```python
from build123d import *

# Parameters (mm, degrees)
CROQUIS1_R              = 2.55
SALIENTE_EXTRUIR1_DEPTH = 400


with BuildPart() as part:
    # Croquis1 → Saliente-Extruir1 (new body)
    with BuildSketch(Plane.XY):
        with BuildLine():
            Line((-20, -9), (-20, -3.95))
            ThreePointArc((-20, -3.95), (-19.912132034, -3.737867966), (-19.7, -3.65))
            Line((-19.7, -3.65), (-19.5, -3.65))
            Line((-19.5, -3.65), (-19.5, -3.15))
            Line((-19.5, -3.15), (-18, -3.15))
            Line((-18, -3.15), (-18, -4.85))
            ThreePointArc((-18, -4.85), (-17.912132034, -5.062132034), (-17.7, -5.15))
            Line((-17.7, -5.15), (-16.5, -5.15))
            Line((-16.5, -5.15), (-14.485786438, -3.135786438))
            ThreePointArc((-14.485786438, -3.135786438), (-14.052240935, -2.48693974), (-13.9, -1.721572875))
            Line((-13.9, -1.721572875), (-13.9, 1.721572875))
            ThreePointArc((-13.9, 1.721572875), (-14.052240935, 2.48693974), (-14.485786438, 3.135786438))
            Line((-14.485786438, 3.135786438), (-16.5, 5.15))
            Line((-16.5, 5.15), (-17.7, 5.15))
            ThreePointArc((-17.7, 5.15), (-17.912132034, 5.062132034), (-18, 4.85))
            Line((-18, 4.85), (-18, 3.15))
            Line((-18, 3.15), (-19.5, 3.15))
            Line((-19.5, 3.15), (-19.5, 3.65))
            Line((-19.5, 3.65), (-19.7, 3.65))
            ThreePointArc((-19.7, 3.65), (-19.912132034, 3.737867966), (-20, 3.95))
            Line((-20, 3.95), (-20, 9))
            ThreePointArc((-20, 9), (-19.707106781, 9.707106781), (-19, 10))
            Line((-19, 10), (-13.95, 10))
            ThreePointArc((-13.95, 10), (-13.737867966, 9.912132034), (-13.65, 9.7))
            Line((-13.65, 9.7), (-13.65, 9.5))
            Line((-13.65, 9.5), (-13.15, 9.5))
            Line((-13.15, 9.5), (-13.15, 8))
            Line((-13.15, 8), (-14.85, 8))
            ThreePointArc((-14.85, 8), (-15.062132034, 7.912132034), (-15.15, 7.7))
            Line((-15.15, 7.7), (-15.15, 6.5))
            Line((-15.15, 6.5), (-13.135786438, 4.485786438))
            ThreePointArc((-13.135786438, 4.485786438), (-12.48693974, 4.052240935), (-11.721572875, 3.9))
            Line((-11.721572875, 3.9), (-8.278427125, 3.9))
            ThreePointArc((-8.278427125, 3.9), (-7.51306026, 4.052240935), (-6.864213562, 4.485786438))
            Line((-6.864213562, 4.485786438), (-4.85, 6.5))
            Line((-4.85, 6.5), (-4.85, 7.7))
            ThreePointArc((-4.85, 7.7), (-4.937867966, 7.912132034), (-5.15, 8))
            Line((-5.15, 8), (-6.85, 8))
            Line((-6.85, 8), (-6.85, 9.5))
            Line((-6.85, 9.5), (-6.35, 9.5))
            Line((-6.35, 9.5), (-6.35, 9.7))
            ThreePointArc((-6.35, 9.7), (-6.262132034, 9.912132034), (-6.05, 10))
            Line((-6.05, 10), (6.05, 10))
            ThreePointArc((6.05, 10), (6.262132034, 9.912132034), (6.35, 9.7))
            Line((6.35, 9.7), (6.35, 9.5))
            Line((6.35, 9.5), (6.85, 9.5))
            Line((6.85, 9.5), (6.85, 8))
            Line((6.85, 8), (5.15, 8))
            ThreePointArc((5.15, 8), (4.937867966, 7.912132034), (4.85, 7.7))
            Line((4.85, 7.7), (4.85, 6.5))
            Line((4.85, 6.5), (6.864213562, 4.485786438))
            ThreePointArc((6.864213562, 4.485786438), (7.51306026, 4.052240935), (8.278427125, 3.9))
            Line((8.278427125, 3.9), (11.721572875, 3.9))
            ThreePointArc((11.721572875, 3.9), (12.48693974, 4.052240935), (13.135786438, 4.485786438))
            Line((13.135786438, 4.485786438), (15.15, 6.5))
            Line((15.15, 6.5), (15.15, 7.7))
            ThreePointArc((15.15, 7.7), (15.062132034, 7.912132034), (14.85, 8))
            Line((14.85, 8), (13.15, 8))
            Line((13.15, 8), (13.15, 9.5))
            Line((13.15, 9.5), (13.65, 9.5))
            Line((13.65, 9.5), (13.65, 9.7))
            ThreePointArc((13.65, 9.7), (13.737867966, 9.912132034), (13.95, 10))
            Line((13.95, 10), (19, 10))
            ThreePointArc((19, 10), (19.707106781, 9.707106781), (20, 9))
            Line((20, 9), (20, 3.95))
            ThreePointArc((20, 3.95), (19.912132034, 3.737867966), (19.7, 3.65))
            Line((19.7, 3.65), (19.5, 3.65))
            Line((19.5, 3.65), (19.5, 3.15))
            Line((19.5, 3.15), (18, 3.15))
            Line((18, 3.15), (18, 4.85))
            ThreePointArc((18, 4.85), (17.912132034, 5.062132034), (17.7, 5.15))
            Line((17.7, 5.15), (16.5, 5.15))
            Line((16.5, 5.15), (14.485786438, 3.135786438))
            ThreePointArc((14.485786438, 3.135786438), (14.052240935, 2.48693974), (13.9, 1.721572875))
            Line((13.9, 1.721572875), (13.9, -1.721572875))
            ThreePointArc((13.9, -1.721572875), (14.052240935, -2.48693974), (14.485786438, -3.135786438))
            Line((14.485786438, -3.135786438), (16.5, -5.15))
            Line((16.5, -5.15), (17.7, -5.15))
            ThreePointArc((17.7, -5.15), (17.912132034, -5.062132034), (18, -4.85))
            Line((18, -4.85), (18, -3.15))
            Line((18, -3.15), (19.5, -3.15))
            Line((19.5, -3.15), (19.5, -3.65))
            Line((19.5, -3.65), (19.7, -3.65))
            ThreePointArc((19.7, -3.65), (19.912132034, -3.737867966), (20, -3.95))
            Line((20, -3.95), (20, -9))
            ThreePointArc((20, -9), (19.707106781, -9.707106781), (19, -10))
            Line((19, -10), (13.65, -10))
            Line((13.65, -10), (13.65, -9.5))
            Line((13.65, -9.5), (13.15, -9.5))
            Line((13.15, -9.5), (13.15, -8))
            Line((13.15, -8), (14.85, -8))
            ThreePointArc((14.85, -8), (15.062132034, -7.912132034), (15.15, -7.7))
            Line((15.15, -7.7), (15.15, -6.5))
            Line((15.15, -6.5), (13.135786438, -4.485786438))
            ThreePointArc((13.135786438, -4.485786438), (12.48693974, -4.052240935), (11.721572875, -3.9))
            Line((11.721572875, -3.9), (8.278427125, -3.9))
            ThreePointArc((8.278427125, -3.9), (7.51306026, -4.052240935), (6.864213562, -4.485786438))
            Line((6.864213562, -4.485786438), (4.85, -6.5))
            Line((4.85, -6.5), (4.85, -7.7))
            ThreePointArc((4.85, -7.7), (4.937867966, -7.912132034), (5.15, -8))
            Line((5.15, -8), (6.85, -8))
            Line((6.85, -8), (6.85, -9.5))
            Line((6.85, -9.5), (6.35, -9.5))
            Line((6.35, -9.5), (6.35, -9.7))
            ThreePointArc((6.35, -9.7), (6.262132034, -9.912132034), (6.05, -10))
            Line((6.05, -10), (0, -10))
            Line((0, -10), (-6.05, -10))
            ThreePointArc((-6.05, -10), (-6.262132034, -9.912132034), (-6.35, -9.7))
            Line((-6.35, -9.7), (-6.35, -9.5))
            Line((-6.35, -9.5), (-6.85, -9.5))
            Line((-6.85, -9.5), (-6.85, -8))
            Line((-6.85, -8), (-5.15, -8))
            ThreePointArc((-5.15, -8), (-4.937867966, -7.912132034), (-4.85, -7.7))
            Line((-4.85, -7.7), (-4.85, -6.5))
            Line((-4.85, -6.5), (-6.864213562, -4.485786438))
            ThreePointArc((-6.864213562, -4.485786438), (-7.51306026, -4.052240935), (-8.278427125, -3.9))
            Line((-8.278427125, -3.9), (-11.721572875, -3.9))
            ThreePointArc((-11.721572875, -3.9), (-12.48693974, -4.052240935), (-13.135786438, -4.485786438))
            Line((-13.135786438, -4.485786438), (-15.15, -6.5))
            Line((-15.15, -6.5), (-15.15, -7.7))
            ThreePointArc((-15.15, -7.7), (-15.062132034, -7.912132034), (-14.85, -8))
            Line((-14.85, -8), (-13.15, -8))
            Line((-13.15, -8), (-13.15, -9.5))
            Line((-13.15, -9.5), (-13.65, -9.5))
            Line((-13.65, -9.5), (-13.65, -9.7))
            ThreePointArc((-13.65, -9.7), (-13.737867966, -9.912132034), (-13.95, -10))
            Line((-13.95, -10), (-19, -10))
            ThreePointArc((-19, -10), (-19.707106781, -9.707106781), (-20, -9))
        make_face()
        with Locations((-10, 0)):
            Circle(CROQUIS1_R, mode=Mode.SUBTRACT)
        with Locations((10, 0)):
            Circle(CROQUIS1_R, mode=Mode.SUBTRACT)
        with BuildLine():
            Line((-6.1, 1.721572875), (-6.1, -1.721572875))
            ThreePointArc((-6.1, -1.721572875), (-5.947759065, -2.48693974), (-5.514213562, -3.135786438))
            Line((-5.514213562, -3.135786438), (-3.5, -5.15))
            Line((-3.5, -5.15), (-0.942893219, -7.707106781))
            ThreePointArc((-0.942893219, -7.707106781), (-0.61846987, -7.923879533), (-0.235786438, -8))
            Line((-0.235786438, -8), (0.235786438, -8))
            ThreePointArc((0.235786438, -8), (0.61846987, -7.923879533), (0.942893219, -7.707106781))
            Line((0.942893219, -7.707106781), (3.5, -5.15))
            Line((3.5, -5.15), (5.514213562, -3.135786438))
            ThreePointArc((5.514213562, -3.135786438), (5.947759065, -2.48693974), (6.1, -1.721572875))
            Line((6.1, -1.721572875), (6.1, 1.721572875))
            ThreePointArc((6.1, 1.721572875), (5.947759065, 2.48693974), (5.514213562, 3.135786438))
            Line((5.514213562, 3.135786438), (3.5, 5.15))
            Line((3.5, 5.15), (0.942893219, 7.707106781))
            ThreePointArc((0.942893219, 7.707106781), (0.61846987, 7.923879533), (0.235786438, 8))
            Line((0.235786438, 8), (-0.235786438, 8))
            ThreePointArc((-0.235786438, 8), (-0.61846987, 7.923879533), (-0.942893219, 7.707106781))
            Line((-0.942893219, 7.707106781), (-3.5, 5.15))
            Line((-3.5, 5.15), (-5.514213562, 3.135786438))
            ThreePointArc((-5.514213562, 3.135786438), (-5.947759065, 2.48693974), (-6.1, 1.721572875))
        make_face(mode=Mode.SUBTRACT)
    extrude(amount=SALIENTE_EXTRUIR1_DEPTH)


solid = part.part
```
Build history of the part. All positions in model axes, mm. Coordinates: 2 decimals unless noted, no trailing zeros.
Item 1: Drop flat-ended pins along their axis: pin 1 Ø1.5 at (x, z) = (9, 277.5) entering from +Y; pin 2 Ø4 at (x, z) = (10, 68) entering from -Y; pin 3 Ø5 at (x, y) = (-0.5, 1.5) entering from +Z; pin 4 Ø0.6 at (y, z) = (-9.5, 209.5) entering from -X. Give the stop position or say it passes through.
Filled in:
pin 1: stops at y = 3.9
pin 2: stops at y = -3.92
pin 3: passes through
pin 4: stops at x = -19.98
Item 2: Saw through at A-A on z = 139. State how many separate pieces and enclosed holes the cut face has, then the cut area to 3 significant figures.
Filled in:
separate pieces: 1
enclosed holes: 3
area: 333 mm2
Item 3: Drill centre lines: L1, parallel to X at y = -8.5, z = 197; L2, parallel to X at y = 0.25, z = 140.5; L3, parallel to Y at x = -15, z = 224. Where is each one in solid material? Low to high.
Filled in:
L1: x = -20 to -13.15, -6.85 to 6.85, 13.15 to 20
L2: x = -13.9 to -12.54, -7.46 to -6.1, 6.1 to 7.46, 12.54 to 13.9
L3: y = -10 to -7.96, -6.35 to -3.65, 3.65 to 6.35, 7.96 to 10
